```python
from build123d import *

# Parameters (mm, degrees)
EXTRUDE_1_DEPTH     = 134.35
SKETCH_2_OUTSIDE_W  = 174.82
SKETCH_2_OUTSIDE_H  = 174.82
CUT_EXTRUDE_1_DEPTH = 193.353437713
CUT_EXTRUDE_START   = -10
CUT_EXTRUDE_2_DEPTH = 10
EXTRUDE_2_DEPTH     = 22.5


# Read off the part's stored shape, not the designer's step: Вырез-Вытянуть2
with BuildPart() as part:
    # Эскиз1 → Бобышка-Вытянуть1 (new body)
    with BuildSketch(Plane.XY):
        Polygon((0, 0), (0, 30), (39.675, 30), (59.675, 10), (74.675, 10), (94.675, 30), (134.35, 30), (134.35, 0), align=None)
    extrude(amount=EXTRUDE_1_DEPTH)

    # Эскиз2 outside → Вырез-Вытянуть1 (cut, through all)
    with BuildSketch(Plane.XZ):
        with Locations((67.175, 67.175)):
            Rectangle(SKETCH_2_OUTSIDE_W, SKETCH_2_OUTSIDE_H)
        Polygon((127.278932188, 134.35), (0, 7.071067812), (7.071067812, 0), (134.35, 127.278932188), align=None, mode=Mode.SUBTRACT)
    extrude(amount=-CUT_EXTRUDE_1_DEPTH, mode=Mode.SUBTRACT)

    # Вырез-Вытянуть2 outline → Вырез-Вытянуть2 (cut)
    with BuildSketch(Plane(origin=(-3.535533906, 0, 3.535533906), x_dir=(0.7071067811865475, 0, 0.7071067811865477), z_dir=(-0.7071067811865477, 0, 0.7071067811865475)).offset(CUT_EXTRUDE_START)):
        with BuildLine():
            Line((5, 30), (5, 3.483288217))
            ThreePointArc((5, 3.483288217), (8.102307967, 12.618107552), (16.125989905, 17.974390514))
            Line((16.125989905, 17.974390514), (61.108923087, 30))
            Line((61.108923087, 30), (5, 30))
        make_face()
        with BuildLine():
            Line((184.999592105, 30), (128.634264977, 30))
            Line((128.634264977, 30), (128.820557467, 29.950423647))
            Line((128.820557467, 29.950423647), (173.857147448, 17.965239064))
            ThreePointArc((173.857147448, 17.965239064), (181.89209668, 12.611319604), (184.999592105, 3.469747807))
            Line((184.999592105, 3.469747807), (184.999592105, 30))
        make_face()
    extrude(amount=CUT_EXTRUDE_2_DEPTH, mode=Mode.SUBTRACT)

    # Эскиз5 → Бобышка-Вытянуть2 (add)
    with BuildSketch(Plane.XZ):
        Polygon((134.35, 127.278932188), (127.278932188, 134.35), (0, 7.071067812), (7.071067812, 0), align=None)
    extrude(amount=EXTRUDE_2_DEPTH)


solid = part.part
```
Geometry check sheet. Reference: the model listing, model coordinates, mm. A direction names the side the tool comes from. Coordinates: 2 decimals unless noted, no trailing zeros. Loops run counter-clockwise (first coordinate to the right, second up) from the corner with the lowest first, then second, coordinate; pieces in that order, holes last. Notation, with made-up numbers: (-39, 87.5) - (-27, 87.5) arc R35 cw to (-27, 123.5) - close; hole circle Ø9 at (-23, -14). An arc over 180 degrees is marked (long way). One line per item, written item: value. Start each with the question number.
(1) Material ranges on line 1 (X direction, y = 6, z = 114.5); line 2 (X direction, y = -3.5, z = 68); line 3 (Z direction, x = 35, y = -19), recorded low to high. Write a range as [from, to].
(2) Cross-section at D-D on y = 14. Enter the section's corners in (x, z) (3 decimals).
(3) Cross-section at A-A on y = 22.5. Enter the section's corners in (x, z) (1 decimal).
(4) Cross-section at C-C on z = 50.5. Enter the section's corners in (x, y).
(5) Depth check by flat-ended pin: P1, Ø1.5, axis at y = -8.5, z = 44.5, coming from the +X side; P2, Ø8, axis at x = 22.5, y = -5, coming from the +Z side; P3, Ø10, axis at x = 92, y = 14.5, coming from the +Z side. Enter the tip coordinate at first touch or a pass-through.
(6) Cross-section at B-B on y = -4. Enter the section's corners in (x, z), plus the area to 3 significant figures.
(7) Tool access check on faces 1 (the flat face through (69.82, -1.74, 62.75)), 2 (the flat face through (67, 10, 67)). Record the directions out of +Z, -Z, +X, -X, +Y, -Y that give a thin tool (end or side, any length) a straight path to the whole face; none if there is none.
Results below:
1. line 1: x = [107.43, 121.57]
1. line 2: x = [60.93, 75.07]
1. line 3: z = [27.93, 42.07]
2. outline: (3.044, 10.115) - (10.115, 3.044) - (55.675, 48.604) - (55.675, 62.746) - close; (78.675, 71.604) - (131.297, 124.226) - (124.226, 131.297) - (78.675, 85.746) - close
3. outline: (19.8, 26.9) - (26.9, 19.8) - (47.2, 40.1) - (47.2, 54.2) - close; (87.2, 80.1) - (114.4, 107.4) - (107.4, 114.4) - (87.2, 94.2) - close
4. outline: (43.43, -22.5) - (57.57, -22.5) - (57.57, 12.1) - (43.43, 26.25) - close
5. P1: stops at x = 52.32
5. P2: stops at z = 33.57
5. P3: stops at z = 104.07
6. outline: (0, 7.07) - (7.07, 0) - (134.35, 127.28) - (127.28, 134.35) - close
6. area: 1,800 mm2
7. face 1: -Z, +X, +Y, -Y
7. face 2: +Z, -Z, +Y
